Input: part model. Units: mm. Frame: model coordinates. Round coordinates to 2 decimals unless told otherwise and drop trailing zeros. Write each loop counter-clockwise with the first axis right and the second up, starting at its lowest first coordinate (ties: lowest second). Pieces come first, ordered by that corner, then holes. Notation, with made-up numbers: M 61.25,29.25 L 105.25,29.25 A25 ccw 105.25,54.25 Z; hole C 12,-13.5 d11. An arc over 180 degrees is marked long. Write each question's results on one line, items separated by ' | '. Start each with the question number.
```python
from build123d import *

# Parameters (mm, degrees)
F1_DEPTH = 3.175


with BuildPart() as f1:
    # F0 (on Front) → F1 (new body, symmetric)
    with BuildSketch(Plane.XZ):
        with BuildLine():
            Line((457.2, 3.4925), (0, 3.4925))
            ThreePointArc((0, 3.4925), (-3.4925, 0), (0, -3.4925))
            ThreePointArc((0, -3.4925), (0.027733, -3.49239), (0.055465, -3.49206))
            Line((0.055465, -3.49206), (457.213318, 0.138283))
            ThreePointArc((457.213318, 0.138283), (458.877122, 1.822024), (457.2, 3.4925))
        make_face()
        with BuildLine():
            ThreePointArc((0.025836, -3.174895), (-3.174974, -0.012918), (0, 3.175))
            Line((0, 3.175), (457.200249, 3.085365))
            ThreePointArc((457.200249, 3.085365), (458.47, 1.81524), (457.2, 0.545365))
            Line((457.2, 0.545365), (0.025836, -3.174895))
        make_face(mode=Mode.SUBTRACT)
    extrude(amount=F1_DEPTH, both=True)


solid = f1.part
```
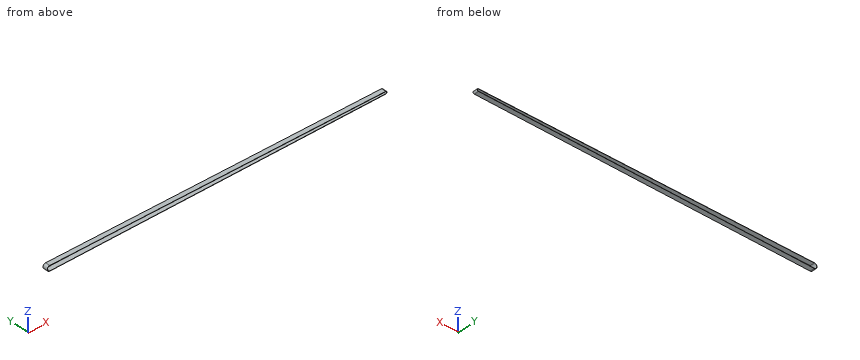
1. Cut plane A-A on z = -2. Output: boundary loops of the cut face in (x, y) (3 decimals).
2. Line query: L1, parallel to Z at x = 328, y = -1.5; L2, parallel to Z at x = 359.5, y = -2.25; L3, parallel to X at y = 1, z = 2.5. Output: solid intervals per line, ascending. Write a range as from..to.
3. Contact query for flat-ended pins moving along their axis: P1, Ø3, axis at x = 83.5, z = 0.5, coming from the +Y side; P2, Ø3, axis at y = -2.5, z = 0, coming from the +X side. Output: stop coordinate, or through.
Answers follow:
1) outline: M -2.863,-3.175 L -2.466,-3.175 L -2.466,3.175 L -2.863,3.175 Z; M 144.406,-3.175 L 187.946,-3.175 L 187.946,3.175 L 144.406,3.175 Z
2) L1: z = -0.89..-0.51, 3.11..3.49 | L2: z = -0.64..-0.25, 3.1..3.49 | L3: x = -2.44..-1.96, 458.27..458.73
3) P1: passes through | P2: stops at x = 458.85
